Check sheet for the modelled part. Datum: model origin and axes. Units: mm. A direction names the side the tool comes from. Coordinates: 2 decimals unless noted, no trailing zeros. Write each loop counter-clockwise with the first axis right and the second up, starting at its lowest first coordinate (ties: lowest second). Pieces come first, ordered by that corner, then holes. Notation, with made-up numbers: (79.25, 32) -> (111.25, 32) arc R9 cw to (111.25, 43) -> close; hole circle Ø2 at (30.25, -12). An arc over 180 degrees is marked (long way). Put each result on its own line as item: value.
```python
from build123d import *

# Parameters (mm, degrees)
F0_W     = 21.43125
F0_H     = 2.38125
F1_DEPTH = 5.55625
F2_R     = 2.778115
F3_R     = 1.2192
F4_DEPTH = 25.4


# Not quite as in the source:
# - a fillet or chamfer is up to 0.001 mm smaller than in the source, because OpenCascade refuses the exact size
# - ends of sketch curves that miss each other by under 0.0002 mm in the source are joined


with BuildPart() as f1:
    # F0 (on Top) → F1 (new body)
    with BuildSketch(Plane.XY):
        with Locations((16.6664377481, 21.9699217558)):
            Rectangle(F0_W, F0_H)
    extrude(amount=F1_DEPTH)

    # F2 (radius 2.778125 in the source; OpenCascade refuses exactly that, so slightly less here)
    f2_edges = [f1.edges().sort_by_distance(p)[0] for p in [
        (27.382063, 21.969922, 5.55625),
        (27.382063, 21.969922, 0),
        (5.950813, 21.969922, 5.55625),
        (5.950813, 21.969922, 0),
    ]]
    fillet(f2_edges, radius=F2_R)

    # F3 (on face) → F4 (cut)
    with BuildSketch(Plane.XZ.offset(-20.7792967558)):
        with Locations((8.7289377481, 2.778125)):
            Circle(F3_R)
        with Locations((24.6039377481, 2.778125)):
            Circle(F3_R)
        with BuildLine():
            Line((24.6039477481, 5.55625), (8.7289277481, 5.55625))
            ThreePointArc((8.7289277481, 5.55625), (9.7548283932, 5.3598931731), (10.6356999108, 4.7985795455))
            ThreePointArc((10.6356999108, 4.7985795455), (11.1390550638, 4.4778289011), (11.7252782896, 4.365625))
            Line((11.7252782896, 4.365625), (21.6075972066, 4.365625))
            ThreePointArc((21.6075972066, 4.365625), (22.1938204324, 4.4778289011), (22.6971755853, 4.7985795455))
            ThreePointArc((22.6971755853, 4.7985795455), (23.5780471029, 5.3598931731), (24.6039477481, 5.55625))
        make_face()
        with BuildLine():
            ThreePointArc((10.6356999108, 0.7576704545), (9.7548283932, 0.1963568269), (8.7289377481, 0))
            Line((8.7289377481, 0), (24.6039477481, 0))
            ThreePointArc((24.6039477481, 0), (23.5780471029, 0.1963568269), (22.6971755853, 0.7576704545))
            ThreePointArc((22.6971755853, 0.7576704545), (22.1938204324, 1.0784210989), (21.6075972066, 1.190625))
            Line((21.6075972066, 1.190625), (11.7252782896, 1.190625))
            ThreePointArc((11.7252782896, 1.190625), (11.1390550638, 1.0784210989), (10.6356999108, 0.7576704545))
        make_face()
    extrude(amount=-F4_DEPTH, mode=Mode.SUBTRACT)


solid = f1.part
```
Q1. Cross-section at D-D (z = 3). Record the cut outline in (x, y), plus the area to 3 significant figures.
Recorded:
outline: (5.96, 20.78) -> (7.53, 20.78) -> (7.53, 23.16) -> (5.96, 23.16) -> close; (9.93, 20.78) -> (23.41, 20.78) -> (23.41, 23.16) -> (9.93, 23.16) -> close; (25.8, 20.78) -> (27.37, 20.78) -> (27.37, 23.16) -> (25.8, 23.16) -> close
area: 39.6 mm2
Q2. Cross-section at C-C (x = 9.75). Record the cut outline in (y, z).
Recorded:
outline: (20.78, 0.19) -> (23.16, 0.19) -> (23.16, 2.11) -> (20.78, 2.11) -> close; (20.78, 3.44) -> (23.16, 3.44) -> (23.16, 5.36) -> (20.78, 5.36) -> close
Q3. Mould release check, pull along Z, two halves, no side actions. Record for faces 1 (the flat face through (17, 22, 4.366)), 2 (the cylindrical face through (11.147, 21.953, 1.082)), 3 (the cylindrical face through (25.77, 21.95, 3.14)): released by +Z, released by -Z, zero draft, split by the parting line, or undercut.
Recorded:
face 1: released by +Z
face 2: released by -Z
face 3: undercut
Q4. Cross-section at B-B (z = 1.8). Record the cut outline in (x, y).
Recorded:
outline: (6.13, 20.78) -> (8, 20.78) -> (8, 23.16) -> (6.13, 23.16) -> close; (9.46, 20.78) -> (23.88, 20.78) -> (23.88, 23.16) -> (9.46, 23.16) -> close; (25.33, 20.78) -> (27.2, 20.78) -> (27.2, 23.16) -> (25.33, 23.16) -> close
Q5. Depth check by flat-ended pin: P1, Ø1, axis at x = 20, y = 21.5, coming from the -Z side; P2, Ø1.2, axis at x = 19, y = 22, coming from the +Z side. Enter the tip coordinate at first touch or a pass-through.
Recorded:
P1: stops at z = 1.19
P2: stops at z = 4.37
Q6. Material ranges on line 1 along X through (y, z) = (22.6, 2.85); line 2 along Z through (x, y) = (8.75, 21.3); line 3 along X through (y, z) = (22.55, 2.35), recorded low to high.
Recorded:
line 1: x = 5.95 to 7.51, 9.95 to 23.39, 25.82 to 27.38
line 2: z = 0 to 1.56, 4 to 5.56
line 3: x = 5.98 to 7.59, 9.87 to 23.46, 25.75 to 27.35
Q7. Cross-section at A-A (y = 21.9). State how many separate pieces and enclosed holes the cut face has, plus the area to 3 significant figures.
Recorded:
separate pieces: 1
enclosed holes: 2
area: 73.2 mm2
Q8. Tool access check on faces 4 (the cylindrical face through (23.59, 21.95, 0.19)), 5 (the cylindrical face through (6.74, 21.99, 4.72)), 6 (the cylindrical face through (22.186, 21.953, 4.475)). Record the directions out of +Z, -Z, +X, -X, +Y, -Y that give a thin tool (end or side, any length) a straight path to the whole face; none if there is none.
Recorded:
face 4: -Z, +Y, -Y
face 5: +Z, -X, +Y, -Y
face 6: +Z, +Y, -Y
